CAD build for the part. Positions are in the model's coordinates, mm. A direction names the side the tool comes from. Round coordinates to 2 decimals unless told otherwise and drop trailing zeros. Write each loop counter-clockwise with the first axis right and the second up, starting at its lowest first coordinate (ties: lowest second). Pieces come first, ordered by that corner, then holes. Notation, with made-up numbers: M 29.25,48 L 81.25,48 A27 cw 81.25,78 Z; hole C 68.25,84.5 d1. An arc over 180 degrees is marked long. Write each question's results on one line, items separated by ' | '. Start each with the question number.
```python
from build123d import *

# Parameters (mm, degrees)
RESSALTO_EXTRUS_O1_DEPTH = 12.5
RESSALTO_EXTRUS_O2_DEPTH = 5.8
CORTE_EXTRUS_O1_DEPTH    = 5.5
ESBO_O4_R                = 2.25
RESSALTO_EXTRUS_O3_DEPTH = 4


with BuildPart() as part:
    # Esboço1 → Ressalto-extrusão1 (new body)
    with BuildSketch(Plane.XY):
        Polygon((11.35, 11.75), (15.95, 11.75), (15.95, 9.15), (11.35, 9.15), (11.35, -9.15), (-11.35, -9.15), (-11.35, 9.15), (-15.95, 9.15), (-15.95, 11.75), (-11.35, 11.75), (-11.35, 12.95), (11.35, 12.95), align=None)
    extrude(amount=RESSALTO_EXTRUS_O1_DEPTH)

    # Esboço2 → Ressalto-extrusão2 (add)
    with BuildSketch(Plane(origin=(0, 12.95, 0), x_dir=(1, 0, 0), z_dir=(0, 1, 0))):
        with BuildLine():
            ThreePointArc((-0.394078947, -4.04425888), (-11.35, -6.25), (-0.394078947, -8.45574112))
            ThreePointArc((-0.394078947, -8.45574112), (2.3, -6.25), (-0.394078947, -4.04425888))
        make_face()
    extrude(amount=RESSALTO_EXTRUS_O2_DEPTH)

    # Esboço3 → Corte-extrusão1 (cut)
    with BuildSketch(Plane(origin=(0, 11.75, 0), x_dir=(1, 0, 0), z_dir=(0, 1, 0))):
        with BuildLine():
            Line((-15.95, -7.25), (-14.679795897, -7.25))
            ThreePointArc((-14.679795897, -7.25), (-12.3, -6.25), (-14.679795897, -5.25))
            Line((-14.679795897, -5.25), (-15.95, -5.25))
            Line((-15.95, -5.25), (-15.95, -7.25))
        make_face()
        with BuildLine():
            Line((15.95, -5.25), (15.95, -7.25))
            Line((15.95, -7.25), (14.679795897, -7.25))
            ThreePointArc((14.679795897, -7.25), (12.3, -6.25), (14.679795897, -5.25))
            Line((14.679795897, -5.25), (15.95, -5.25))
        make_face()
    extrude(amount=-CORTE_EXTRUS_O1_DEPTH, mode=Mode.SUBTRACT)

    # Esboço4 → Ressalto-extrusão3 (add)
    with BuildSketch(Plane(origin=(0, 18.75, 0), x_dir=(1, 0, 0), z_dir=(0, 1, 0))):
        with Locations(Location((-5.65, -6.25, 0), (0, 0, 270))):
            Circle(ESBO_O4_R)
    extrude(amount=RESSALTO_EXTRUS_O3_DEPTH)


solid = part.part
```
1) 3-axis set-ups, long thin cutter, end or side, ignore diameter. For faces 5 (the face through (-3, 18.75, 6)), 6 (the face through (11.35, 0, 6)), 7 (the face through (-13.17, 11.75, 4.77)): which of +Z, -Z, +X, -X, +Y, -Y reach the whole face in a straight line?
2) Saw through at C-C, the plane z = 9. Write the cut outline in (x, y).
3) Drop flat-ended pins along their axis: pin 1 Ø6 at (y, z) = (16.5, 9.5) entering from +X; pin 2 Ø1.3 at (y, z) = (12.5, 6.5) entering from -X; pin 3 Ø3.5 at (x, z) = (-14, 6.5) entering from +Y; pin 4 Ø1.4 at (x, z) = (14.5, 6.5) entering from +Y. Give the stop position or say it passes through.
4) Pull direction Z, two halves, no side cores. Call faces 1 (the face through (0, 2, 12.5)), 2 (the face through (-4.974, 20.722, 8.396)), 3 (the face through (-12.3, 10.5, 6.3)), 4 (the face through (11.35, 12, 6)): pulls with the +Z half, pulls with the -Z half, needs draft (parallel to the pull), parting line crosses it, or undercut.
5) Saw through at D-D, the plane y = -4.5. Write the cut outline in (x, z).
6) Saw through at B-B, the plane x = 0.05. Write the cut outline in (y, z), plus the area to 3 significant figures.
7) Saw through at A-A, the plane x = 13.7. Write the cut outline in (y, z).
8) Wall check: line 1 along Z through (x, y) = (-13.7, 9.9); line 2 along Y through (x, z) = (-5, 1.5); line 3 along Y through (x, z) = (-11, 3.25). Give the ranges that are in metal, low to high. Write a range as from..to.
Filled sheet:
1) face 5: +Y | face 6: +Z, -Z, +X, -Y | face 7: +Z, -Z, -X, +Y
2) outline: M -15.95,9.15 L -11.35,9.15 L -11.35,-9.15 L 11.35,-9.15 L 11.35,9.15 L 15.95,9.15 L 15.95,11.75 L 11.35,11.75 L 11.35,12.95 L -0.66,12.95 L -0.66,18.75 L -10.64,18.75 L -10.64,12.95 L -11.35,12.95 L -11.35,11.75 L -15.95,11.75 Z
3) pin 1: stops at x = 2.29 | pin 2: stops at x = -11.35 | pin 3: stops at y = 11.75 | pin 4: passes through
4) face 1: pulls with the +Z half | face 2: parting line crosses it | face 3: undercut | face 4: needs draft
5) outline: M -11.35,0 L 11.35,0 L 11.35,12.5 L -11.35,12.5 Z
6) outline: M -9.15,0 L 12.95,0 L 12.95,4 L 18.75,4 L 18.75,8.5 L 12.95,8.5 L 12.95,12.5 L -9.15,12.5 Z | area: 302 mm^2
7) outline: M 9.15,0 L 11.75,0 L 11.75,4.85 L 9.15,4.85 Z; M 9.15,7.65 L 11.75,7.65 L 11.75,12.5 L 9.15,12.5 Z
8) line 1: z = 0..4.85, 7.65..12.5 | line 2: y = -9.15..18.75 | line 3: y = -9.15..12.95
